Geometry check sheet. Reference: the model listing, model coordinates, mm. A direction names the side the tool comes from. Coordinates: 2 decimals unless noted, no trailing zeros. Write each loop counter-clockwise with the first axis right and the second up, starting at its lowest first coordinate (ties: lowest second). Pieces come first, ordered by that corner, then holes. Notation, with made-up numbers: (86, -16) -> (95, -16) arc R25 ccw to (95, 2) -> close; hole circle Ø2 at (25, 38). An arc over 180 degrees is marked (long way). One line per question, with ' | ' between items.
```python
from build123d import *

# Parameters (mm, degrees)
SKETCH1_R           = 1.1
SKETCH1_R_2         = 0.15
BOSS_EXTRUDE1_DEPTH = 7
SKETCH2_R           = 4
SKETCH2_R_2         = 1.1
BOSS_EXTRUDE2_DEPTH = 0.2
CHAMFER1_SIZE       = 0.2


with BuildPart() as part:
    # Sketch1 → Boss-Extrude1 (new body)
    with BuildSketch(Plane.XY):
        Circle(SKETCH1_R)
        Circle(SKETCH1_R_2, mode=Mode.SUBTRACT)
    extrude(amount=BOSS_EXTRUDE1_DEPTH)

    # Sketch2 → Boss-Extrude2 (add)
    with BuildSketch(Plane.XY.offset(7)):
        with Locations((0.018669882, 0)):
            Circle(SKETCH2_R)
        Circle(SKETCH2_R_2, mode=Mode.SUBTRACT)
    extrude(amount=-BOSS_EXTRUDE2_DEPTH)

    # Chamfer1
    chamfer1_edges = [part.edges().sort_by_distance(p)[0] for p in [
        (-1.1, 0, 0),
        (-0.15, 0, 0),
        (-0.15, 0, 7),
    ]]
    chamfer(chamfer1_edges, length=CHAMFER1_SIZE)


solid = part.part
```
(1) Cross-section at A-A (y = 0). Record the cut outline in (x, z).
Answers below:
outline: (-3.98, 6.8) -> (-1.1, 6.8) -> (-1.1, 0.2) -> (-0.9, 0) -> (-0.35, 0) -> (-0.15, 0.2) -> (-0.15, 6.8) -> (-0.35, 7) -> (-3.98, 7) -> close; (0.15, 0.2) -> (0.35, 0) -> (0.9, 0) -> (1.1, 0.2) -> (1.1, 6.8) -> (4.02, 6.8) -> (4.02, 7) -> (0.35, 7) -> (0.15, 6.8) -> close
(2) Tool access check on faces 1 (the face through (0, -1, 7)), 2 (the face through (1.05, 0.33, 3.45)). Record the directions out of +Z, -Z, +X, -X, +Y, -Y that give a thin tool (end or side, any length) a straight path to the whole face; none if there is none.
Answers below:
face 1: +Z, +X, -X, +Y, -Y | face 2: -Z
(3) Cross-section at C-C (z = 1.5). Record the cut outline in (x, y), plus the area to 3 significant figures.
Answers below:
outline: circle Ø2.2 at (0, 0); hole circle Ø0.3 at (0, 0) | area: 3.73 mm²
(4) Cross-section at B-B (x = 0). Record the cut outline in (y, z).
Answers below:
outline: (-4, 6.8) -> (-1.1, 6.8) -> (-1.1, 0.2) -> (-0.9, 0) -> (-0.35, 0) -> (-0.15, 0.2) -> (-0.15, 6.8) -> (-0.35, 7) -> (-4, 7) -> close; (0.15, 0.2) -> (0.35, 0) -> (0.9, 0) -> (1.1, 0.2) -> (1.1, 6.8) -> (4, 6.8) -> (4, 7) -> (0.35, 7) -> (0.15, 6.8) -> close
(5) Cross-section at D-D (x = 1.75). Record the cut outline in (y, z), plus the area to 3 significant figures.
Answers below:
outline: (-3.61, 6.8) -> (3.61, 6.8) -> (3.61, 7) -> (-3.61, 7) -> close | area: 1.44 mm²
(6) Material ranges on line 1 (Y direction, x = 0, z = 2.5); line 2 (Z direction, x = 2.75, y = -2.5); line 3 (X direction, y = -0.75, z = 5.5), recorded low to high.
Answers below:
line 1: y = -1.1 to -0.15, 0.15 to 1.1 | line 2: z = 6.8 to 7 | line 3: x = -0.8 to 0.8
(7) Depth check by flat-ended pin: P1, Ø4, axis at x = 0, z = 2.5, coming from the +Y side; P2, Ø2.5, axis at x = 2, y = -2, coming from the -Z side; P3, Ø1.5, axis at y = 1, z = 1.5, coming from the +X side. Enter the tip coordinate at first touch or a pass-through.
Answers below:
P1: stops at y = 1.1 | P2: stops at z = 6.8 | P3: stops at x = 1.07
